Check sheet for the modelled part. Datum: model origin and axes. Units: mm. Give positions to 0.01 mm unless a question says otherwise; leave off trailing zeros. Order: outer loops, then holes, each group sorted by start corner. A loop starts at its lowest first (then second) coordinate and runs counter-clockwise, first axis right, second up.
```python
from build123d import *

# Parameters (mm, degrees)
BOSS_EXTRUDE1_DEPTH   = 5.08
F_6_CLEARANCE_HOLE1_D = 3.7973


with BuildPart() as part:
    # Sketch1 → Boss-Extrude1 (new body)
    with BuildSketch(Plane.XY):
        Polygon((0, 0), (228.6, 0), (228.6, 88.9), (88.9, 190.5), (0, 190.5), align=None)
    extrude(amount=BOSS_EXTRUDE1_DEPTH)

    # #6 Clearance Hole1 (through all)
    with Locations(Plane.XY.offset(5.08)):
        with Locations((209.55, 19.05), (19.05, 171.45), (69.85, 171.45), (69.85, 19.05), (19.05, 19.05), (107.95, 19.05), (107.95, 69.85), (209.55, 69.85)):
            Hole(F_6_CLEARANCE_HOLE1_D / 2)


solid = part.part
```
(1) Material ranges on L1, parallel to Y at x = 69.85, z = 2.55; L2, parallel to Y at x = 107.95, z = 1.9; L3, parallel to X at y = 92, z = 4.55, recorded low to high.
Response values:
L1: y = 0 to 17.15, 20.95 to 169.55, 173.35 to 190.5
L2: y = 0 to 17.15, 20.95 to 67.95, 71.75 to 176.65
L3: x = 0 to 224.34
(2) Gauge pin test, flat end, axial feed: pin 1 Ø1 at (y, z) = (165, 2.5) entering from +X. Record the tip position at first contact, or that the pin passes through.
Response values:
pin 1: stops at x = 124.65
(3) Cross-section at B-B on y = 140. Enter the section's corners in (x, z).
Response values:
outline: (0, 0) - (158.34, 0) - (158.34, 5.08) - (0, 5.08) - close
(4) Cross-section at C-C on x = 167.5. Enter the section's corners in (y, z).
Response values:
outline: (0, 0) - (133.34, 0) - (133.34, 5.08) - (0, 5.08) - close
(5) Cross-section at A-A on z = 1.4. Count the separate pieces of the cut face and the enclosed holes in it, then the cut area to 3 significant figures.
Response values:
separate pieces: 1
enclosed holes: 8
area: 36,400 mm2
